```python
from build123d import *

# Parameters (mm, degrees)
SKETCH_5_R          = 3.4
EXTRUDE_2_DEPTH     = 0.8
EXTRUDE_2_2_DEPTH   = 0.8
SKETCH_6_W          = 2.031950572
SKETCH_6_H          = 7.518912136
EXTRUDE_3_DEPTH     = 0.8
SKETCH_7_R          = 2.7
EXTRUDE_4_DEPTH     = 2.8
SKETCH_8_R          = 1.4
EXTRUDE_5_DEPTH     = 1.6
SKETCH_9_W          = 4.279769968
SKETCH_9_H          = 23.306699104
CUT_EXTRUDE_1_DEPTH = 0.8


with BuildPart() as part:
    # Sketch 5 → Extrude 2 (new body)
    with BuildSketch(Plane.XY):
        with Locations((0.12672506, -6)):
            Circle(SKETCH_5_R)
    extrude(amount=EXTRUDE_2_DEPTH)



with BuildPart() as body_2:
    # Sketch 5 → Extrude 2 2 (new body)
    with BuildSketch(Plane.XY):
        Polygon((-3.566095263, 9.4), (3.819545383, 9.4), (0.12672506, 3.003847577), align=None)
    extrude(amount=EXTRUDE_2_2_DEPTH)


with BuildPart() as part_1:
    add(part.part)

    add(body_2.part)  # Extrude 3 merges body 2
    # Sketch 6 → Extrude 3 (add)
    with BuildSketch(Plane(origin=(0, 0, 0), x_dir=(-1, 0, 0), z_dir=(0, 0, -1))):
        with Locations((-0.12672506, 1.004112324)):
            Rectangle(SKETCH_6_W, SKETCH_6_H)
    extrude(amount=-EXTRUDE_3_DEPTH)

    # Sketch 7 → Extrude 4 (add)
    with BuildSketch(Plane(origin=(0, 0, 0), x_dir=(-1, 0, 0), z_dir=(0, 0, -1))):
        with Locations((-0.12672506, -6)):
            Circle(SKETCH_7_R)
        Polygon((-2.607109818, 8.7), (2.353659698, 8.7), (-0.12672506, 4.403847577), align=None)
    extrude(amount=EXTRUDE_4_DEPTH)

    # Sketch 8 → Extrude 5 (add)
    with BuildSketch(Plane.XY.offset(0.8)):
        with Locations((0.12672506, 8)):
            Circle(SKETCH_8_R)
        with Locations((0.12672506, -8)):
            Circle(SKETCH_8_R)
    extrude(amount=EXTRUDE_5_DEPTH)

    # Sketch 9 → Cut-Extrude 1 (cut)
    with BuildSketch(Plane.XY.offset(0.8)):
        with Locations((-4.966610044, 0.180472228)):
            Rectangle(SKETCH_9_W, SKETCH_9_H)
    extrude(amount=-CUT_EXTRUDE_1_DEPTH, mode=Mode.SUBTRACT)


solid = part_1.part
```
Work out the finished part from the listing and answer in its coordinate system (mm). A direction names the side the tool comes from. Give positions to 0.01 mm unless a question says otherwise; leave off trailing zeros. Loops run counter-clockwise (first coordinate to the right, second up) from the corner with the lowest first, then second, coordinate; pieces in that order, holes last. Notation, with made-up numbers: (80, 48) -> (112, 48) arc R17 cw to (112, 59) -> close; hole circle Ø1 at (85.25, 80). An arc over 180 degrees is marked (long way). Use CSV: the item, a comma, the result in double quotes.
1. The part is cut by section C-C (x = -1.5). Write down the section's boundary in (y, z), then the cut area to 3 significant figures.
Found:
outline,"(-8.99, 0) -> (-8.15, 0) -> (-8.15, -2.8) -> (-3.85, -2.8) -> (-3.85, 0) -> (-3.01, 0) -> (-3.01, 0.8) -> (-8.99, 0.8) -> close; (5.82, 0) -> (7.22, 0) -> (7.22, -2.8) -> (8.7, -2.8) -> (8.7, 0) -> (9.4, 0) -> (9.4, 0.8) -> (5.82, 0.8) -> close"
area,"23.8 mm^2"
2. The mould has two halves that part along Y. Classify faces 5 (the cylindrical face through (0.712, -8.636, -1.38)), 6 (the flat face through (0, 8, 2.4)), 7 (the flat face through (0, 8.7, -1)): +Y half, -Y half, draft (parallel to the pull), parting line (faces both ways), or undercut.
Found:
face 5,"undercut"
face 6,"draft"
face 7,"+Y half"
3. The part is cut by section A-A (z = -0.2). Write down the section's boundary in (x, y), then the cut area to 3 significant figures.
Found:
outline,"circle Ø5.4 at (0.13, -6); (-2.35, 8.7) -> (0.13, 4.4) -> (2.61, 8.7) -> close"
area,"33.6 mm^2"
4. Straight lines are drawn through the part: line 1 (Z direction, x = 0.25, y = -2); line 2 (Y direction, x = 0, z = 1.9); line 3 (Y direction, x = -1.5, z = -1.25). For each, find the intervals that lie inside material, in ascending order.
Found:
line 1,"0 to 0.8"
line 2,"-9.39 to -6.61, 6.61 to 9.39"
line 3,"-8.15 to -3.85, 7.22 to 8.7"
5. A tool of negligible diameter and unlimited length cuts with its end or side. For faces 1 (the flat face through (1.35, 6.52, -1.38)), 2 (the cylindrical face through (-0.177, 6.633, 1.589)), 3 (the flat face through (-1.844, 6.418, 0.394)), 4 (the flat face through (2.5, 7.114, 0.394)), from which of +Z, -Z, +X, -X, +Y, -Y can it reach the whole face along a straight path? Write none if from no direction.
Found:
face 1,"-Z, +X"
face 2,"+Z"
face 3,"+Z, -Z, -X"
face 4,"+Z, -Z, +X"
6. Flat-ended cylindrical pins translate along their axes: pin 1 Ø0.8 at (x, z) = (0.5, -1) entering from +Y; pin 2 Ø1 at (y, z) = (5.5, 1) entering from +X; pin 3 Ø0.6 at (y, z) = (1.5, 0.5) entering from -X; pin 4 Ø2 at (x, y) = (-2, 3.5) entering from +Z. Find the tip coordinate at first contact, or state that the pin passes through.
Found:
pin 1,"y = 8.7"
pin 2,"x = 1.83"
pin 3,"x = -0.89"
pin 4,"through"
7. The part is cut by section B-B (y = -6). Write down the section's boundary in (x, z), then the cut area to 3 significant figures.
Found:
outline,"(-2.83, 0) -> (-2.57, 0) -> (-2.57, -2.8) -> (2.83, -2.8) -> (2.83, 0) -> (3.53, 0) -> (3.53, 0.8) -> (-2.83, 0.8) -> close"
area,"20.2 mm^2"
